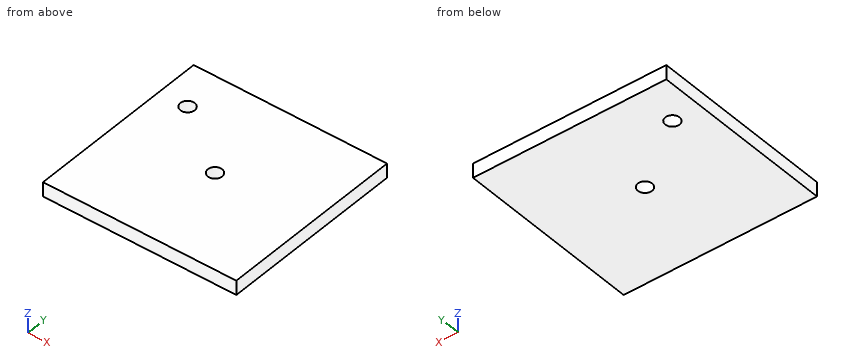
```python
from build123d import *

# Parameters (mm, degrees)
F0_W     = 342.9
F0_H     = 330.2
F1_DEPTH = 25.4
F2_R     = 12.7
F3_DEPTH = 25.401
F4_R     = 12.7
F5_DEPTH = 25.401


with BuildPart() as f1:
    # F0 (on Top) → F1 (new body)
    with BuildSketch(Plane.XY):
        with Locations((171.45, 165.1)):
            Rectangle(F0_W, F0_H)
    extrude(amount=F1_DEPTH)

    # F2 (on face) → F3 (cut, through all)
    with BuildSketch(Plane.XY.offset(25.4)):
        with Locations((50.8, 254)):
            Circle(F2_R)
    extrude(amount=-F3_DEPTH, mode=Mode.SUBTRACT)

    # F4 (on face) → F5 (cut, through all)
    with BuildSketch(Plane.XY.offset(25.4)):
        with Locations((171.45, 165.1)):
            Circle(F4_R)
    extrude(amount=-F5_DEPTH, mode=Mode.SUBTRACT)


solid = f1.part
```
Geometry check sheet. Reference: the model listing, model coordinates, mm. Coordinates: 2 decimals unless noted, no trailing zeros. Write each loop counter-clockwise with the first axis right and the second up, starting at its lowest first coordinate (ties: lowest second). Pieces come first, ordered by that corner, then holes. Notation, with made-up numbers: M 78.5,45.5 L 124.5,45.5 A21 ccw 124.5,53.5 Z; hole C 65,39.25 d5. An arc over 180 degrees is marked long. One line per item, written item: value. Start each with the question number.
(1) Depth check by flat-ended pin: pin 1 (15 mm diameter, centred on x = 171.45, y = 165.1, fed in from +Z). Enter the tip coordinate at first touch or a pass-through.
(2) Sectioned sample at B-B, the plane x = 171.45. Enter the section's corners in (y, z).
(3) Sectioned sample at A-A, the plane y = 254. Enter the section's corners in (x, z), and give its area (3 significant figures).
(4) Scan lines: line 1 along Y through (x, z) = (51, 17.75); line 2 along Y through (x, z) = (171.45, 8.5). Record each from-to range of solid material in increasing order. Write a range as [from, to].
Filled sheet:
1. pin 1: through
2. outline: M 0,0 L 152.4,0 L 152.4,25.4 L 0,25.4 Z; M 177.8,0 L 330.2,0 L 330.2,25.4 L 177.8,25.4 Z
3. outline: M 0,0 L 38.1,0 L 38.1,25.4 L 0,25.4 Z; M 63.5,0 L 342.9,0 L 342.9,25.4 L 63.5,25.4 Z
3. area: 8,060 mm²
4. line 1: [0, 241.3], [266.7, 330.2]
4. line 2: [0, 152.4], [177.8, 330.2]
